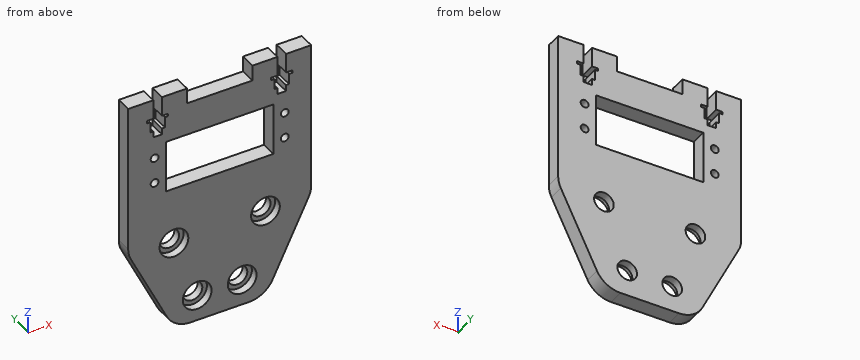
from build123d import *

# Parameters (mm, degrees)
SKETCH1_R           = 1.5
SKETCH1_R_2         = 5.5
SKETCH1_R_3         = 3.75
BOSS_EXTRUDE1_DEPTH = 6
FILLET1_R           = 10
BOSS_EXTRUDE2_START = 3
SKETCH1_3_R         = 5.5
SKETCH1_3_R_2       = 3.75
BOSS_EXTRUDE2_DEPTH = 3
SKETCH1_4_W         = 41
SKETCH1_4_H         = 20
CUT_EXTRUDE2_DEPTH  = 10
SKETCH4_W           = 3.3
SKETCH4_H           = 15
SKETCH4_W_2         = 5.6
SKETCH4_H_2         = 4.1
SKETCH4_W_3         = 8.1
SKETCH4_H_3         = 1
CUT_EXTRUDE3_DEPTH  = 10


with BuildPart() as part:
    # Sketch1 → Boss-Extrude1 (new body)
    with BuildSketch(Plane(origin=(0, 0, 0), x_dir=(1, 0, 0), z_dir=(0, 1, 0))):
        Polygon((17.441626812, 0.78), (-17.441626812, 0.78), (-35, -35.22), (-35, -94.22), (-12.5, -94.22), (-12.5, -88.22), (12.5, -88.22), (12.5, -94.22), (35, -94.22), (35, -35.22), align=None)
        with Locations(Location((-24.889613301, -70.60075616, 0), (0, 0, 270))):
            Circle(SKETCH1_R, mode=Mode.SUBTRACT)
        with Locations(Location((-24.889613301, -60.60075616, 0), (0, 0, 270))):
            Circle(SKETCH1_R, mode=Mode.SUBTRACT)
        with Locations(Location((24.889613301, -70.60075616, 0), (0, 0, 270))):
            Circle(SKETCH1_R, mode=Mode.SUBTRACT)
        with Locations(Location((24.889613301, -60.60075616, 0), (0, 0, 270))):
            Circle(SKETCH1_R, mode=Mode.SUBTRACT)
        with Locations(Location((-17.5, -33.65200814, 0), (0, 0, 270))):
            Circle(SKETCH1_R_2, mode=Mode.SUBTRACT)
        with Locations(Location((-8.607476274, -9.22, 0), (0, 0, 270))):
            Circle(SKETCH1_R_2, mode=Mode.SUBTRACT)
        with Locations(Location((17.5, -33.65200814, 0), (0, 0, 270))):
            Circle(SKETCH1_R_2, mode=Mode.SUBTRACT)
        with Locations(Location((8.607476274, -9.22, 0), (0, 0, 270))):
            Circle(SKETCH1_R_2, mode=Mode.SUBTRACT)
        with Locations(Location((10.3, -65.60075616, 0), (0, 0, 270))):
            Circle(SKETCH1_R_3, mode=Mode.SUBTRACT)
    extrude(amount=BOSS_EXTRUDE1_DEPTH)

    # Fillet1
    fillet1_edges = [part.edges().sort_by_distance(p)[0] for p in [
        (-35, 3, 35.22),
        (-17.441626812, 3, -0.78),
        (17.441626812, 3, -0.78),
        (35, 3, 35.22),
    ]]
    fillet(fillet1_edges, radius=FILLET1_R)

    # Sketch1<3> → Boss-Extrude2 (add)
    # profile 1 of 4: a face of its own
    with BuildSketch(Plane(origin=(0, 0, 0), x_dir=(1, 0, 0), z_dir=(0, 1, 0)).offset(BOSS_EXTRUDE2_START)):
        with Locations(Location((-17.5, -33.65200814, 0), (0, 0, 270))):
            Circle(SKETCH1_3_R)
        with Locations(Location((-17.5, -33.65200814, 0), (0, 0, 270))):
            Circle(SKETCH1_3_R_2, mode=Mode.SUBTRACT)
    # profile 2 of 4: a face of its own
    with BuildSketch(Plane(origin=(0, 0, 0), x_dir=(1, 0, 0), z_dir=(0, 1, 0)).offset(BOSS_EXTRUDE2_START)):
        with Locations(Location((-8.607476274, -9.22, 0), (0, 0, 270))):
            Circle(SKETCH1_3_R)
        with Locations(Location((-8.607476274, -9.22, 0), (0, 0, 270))):
            Circle(SKETCH1_3_R_2, mode=Mode.SUBTRACT)
    # profile 3 of 4: a face of its own
    with BuildSketch(Plane(origin=(0, 0, 0), x_dir=(1, 0, 0), z_dir=(0, 1, 0)).offset(BOSS_EXTRUDE2_START)):
        with Locations(Location((17.5, -33.65200814, 0), (0, 0, 270))):
            Circle(SKETCH1_3_R)
        with Locations(Location((17.5, -33.65200814, 0), (0, 0, 270))):
            Circle(SKETCH1_3_R_2, mode=Mode.SUBTRACT)
    # profile 4 of 4: a face of its own
    with BuildSketch(Plane(origin=(0, 0, 0), x_dir=(1, 0, 0), z_dir=(0, 1, 0)).offset(BOSS_EXTRUDE2_START)):
        with Locations(Location((8.607476274, -9.22, 0), (0, 0, 270))):
            Circle(SKETCH1_3_R)
        with Locations(Location((8.607476274, -9.22, 0), (0, 0, 270))):
            Circle(SKETCH1_3_R_2, mode=Mode.SUBTRACT)
    extrude(amount=BOSS_EXTRUDE2_DEPTH)

    # Sketch1<4> → Cut-Extrude2 (cut)
    with BuildSketch(Plane(origin=(0, 0, 0), x_dir=(1, 0, 0), z_dir=(0, 1, 0))):
        with Locations((0, -65.60075616)):
            Rectangle(SKETCH1_4_W, SKETCH1_4_H)
    extrude(amount=CUT_EXTRUDE2_DEPTH, mode=Mode.SUBTRACT)

    # Sketch4 → Cut-Extrude3 (cut)
    with BuildSketch(Plane.XZ):
        with Locations((-23.75, 86.72)):
            Rectangle(SKETCH4_W, SKETCH4_H)
        with Locations((-23.75, 83.67)):
            Rectangle(SKETCH4_W_2, SKETCH4_H_2)
        with Locations((-23.75, 86.22)):
            Rectangle(SKETCH4_W_3, SKETCH4_H_3)
    cut_extrude3 = extrude(amount=-CUT_EXTRUDE3_DEPTH, mode=Mode.SUBTRACT)

    # Mirror1: Cut-Extrude3 across plane
    add(cut_extrude3.mirror(Plane(origin=(0, 0, 0), x_dir=(0, 0, 1), z_dir=(1, 0, 0))), mode=Mode.SUBTRACT)


solid = part.part
The model under review builds one solid part; all positions refer to its coordinate system, in mm. Round coordinates to 2 decimals unless told otherwise and drop trailing zeros. Write each loop counter-clockwise with the first axis right and the second up, starting at its lowest first coordinate (ties: lowest second). Pieces come first, ordered by that corner, then holes. Notation, with made-up numbers: (62.25, 81) - (90.25, 81) arc R17 ccw to (90.25, 100) - close; hole circle Ø3 at (30.5, 25). An arc over 180 degrees is marked (long way). One line per item, written item: value. Start each with the question number.
1. Consider section B-B on x = -17.5. Write out the cut boundary in (y, z), and give its area (3 significant figures).
2. Consider section D-D on z = 8.5. Write out the cut boundary in (x, y), and give its area (3 significant figures).
3. Clearance check with flat-ended pins moving along their axes: P1, Ø5, axis at x = 15.5, z = 31.5, coming from the -Y side; P2, Ø1.5, axis at y = 5, z = 25.5, coming from the -X side. State where each tip first meets the part, or that it passes through.
4. To check wall thickness, follow L1, parallel to Z at x = -14.5, y = 4.7; L2, parallel to X at y = 2.1, z = 9.22; L3, parallel to X at y = 0.7, z = 10. State the ranges of each line that lie inside material, in increasing order. Write a range as from..to.
5. Consider section A-A on z = 57. Write out the cut boundary in (x, y).
6. Consider section C-C on z = 34.5. Write out the cut boundary in (x, y).
Checks:
1. outline: (0, 1.46) - (6, 1.46) - (6, 29.9) - (3, 29.9) - (3, 28.15) - (0, 28.15) - close; (0, 39.15) - (3, 39.15) - (3, 37.4) - (6, 37.4) - (6, 55.6) - (0, 55.6) - close; (0, 75.6) - (6, 75.6) - (6, 94.22) - (0, 94.22) - close
1. area: 381 mm^2
2. outline: (-21.97, 0) - (-14.06, 0) - (-14.06, 3) - (-12.29, 3) - (-12.29, 6) - (-21.97, 6) - close; (-4.93, 3) - (-3.15, 3) - (-3.15, 0) - (3.15, 0) - (3.15, 3) - (4.93, 3) - (4.93, 6) - (-4.93, 6) - close; (12.29, 3) - (14.06, 3) - (14.06, 0) - (21.97, 0) - (21.97, 6) - (12.29, 6) - close
2. area: 154 mm^2
3. P1: stops at y = 3
3. P2: stops at x = -30.63
4. L1: z = -0.22..31.4, 35.9..55.6, 75.6..94.22
4. L2: x = -22.32..-14.11, -3.11..3.11, 14.11..22.32
4. L3: x = -22.7..-14.05, -3.16..3.16, 14.05..22.7
5. outline: (-35, 0) - (-20.5, 0) - (-20.5, 6) - (-35, 6) - close; (20.5, 0) - (35, 0) - (35, 6) - (20.5, 6) - close
6. outline: (-34.53, 0) - (-22.93, 0) - (-22.93, 3) - (-21.15, 3) - (-21.15, 6) - (-34.53, 6) - close; (-13.85, 3) - (-12.07, 3) - (-12.07, 0) - (12.07, 0) - (12.07, 3) - (13.85, 3) - (13.85, 6) - (-13.85, 6) - close; (21.15, 3) - (22.93, 3) - (22.93, 0) - (34.53, 0) - (34.53, 6) - (21.15, 6) - close
